For this review, use the dimensioned drawing (mm, ordinates from the lowest corner) and the shaded views. A direction names the side the tool comes from. Round coordinates to 2 decimals unless told otherwise and drop trailing zeros. Write each loop counter-clockwise with the first axis right and the second up, starting at its lowest first coordinate (ties: lowest second). Pieces come first, ordered by that corner, then holes. Notation, with made-up numbers: M 73,-39 L 99,-39 A22 cw 99,-1 Z; hole C -39.5,14 d4. An arc over 180 degrees is marked long. Use CSV: the item, a comma, the result in double quotes.
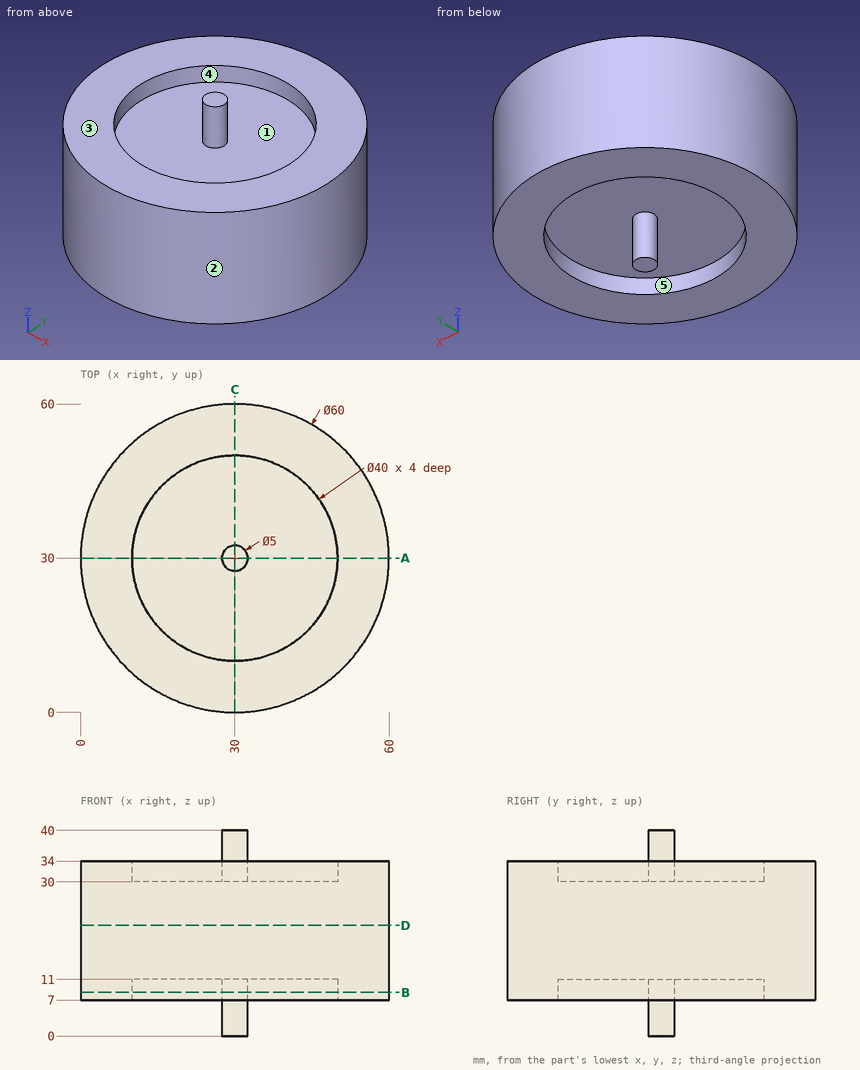
1) Machinability: for the marked faces 4 and 5, which of the approach directions +Z, -Z, +X, -X, +Y, -Y give a long, thin tool a straight path to every point of the face, cutting with its end or side? Answer none if there is none.
Answers:
face 4,"+Z"
face 5,"-Z"
2) Add section A-A on y = 30. Write out the cut boundary in (x, z).
Answers:
outline,"M 0,7 L 10,7 L 10,11 L 27.5,11 L 27.5,0 L 32.5,0 L 32.5,11 L 50,11 L 50,7 L 60,7 L 60,34 L 50,34 L 50,30 L 32.5,30 L 32.5,40 L 27.5,40 L 27.5,30 L 10,30 L 10,34 L 0,34 Z"
3) Add section D-D on z = 21.5. Write out the cut boundary in (x, y), then the cut area to 3 significant figures.
Answers:
outline,"C 30,30 d60"
area,"2,830 mm²"
4) The part is to be moulded in two halves that separate along Y. For the marked faces 1, 2 and 3, say which applies: released by +Y, released by -Y, zero draft, split by the parting line, or undercut.
Answers:
face 1,"undercut"
face 2,"split by the parting line"
face 3,"zero draft"
5) For pin 1 Ø12 at (x, z) = (25.5, 9.5) entering from +Y; pin 2 Ø6 at (y, z) = (41.5, 25) entering from +X; pin 3 Ø18 at (x, y) = (24, 42) entering from -Z; pin 4 Ø1 at (x, z) = (18.5, 6) entering from -Y, all flat-tipped, find the tip position at first contact; note any pin that passes through.
Answers:
pin 1,"y = 60"
pin 2,"x = 58.77"
pin 3,"z = 7"
pin 4,"through"
6) Wall thickness on line 1 along Y through (x, z) = (30, 8.6); line 2 along Z through (x, y) = (29.5, 38.5); line 3 along Z through (x, y) = (4.5, 17): over which ranges is each line inside the solid? List them lowest first. Write a range as [from, to].
Answers:
line 1,"[0, 10], [27.5, 32.5], [50, 60]"
line 2,"[11, 30]"
line 3,"[7, 34]"
7) Add section B-B on z = 8.5. Write out the cut boundary in (x, y), then the cut area to 3 significant figures.
Answers:
outline,"C 30,30 d60; C 30,30 d5; hole C 30,30 d40"
area,"1,590 mm²"
